The listing builds one solid part. Answer for the finished solid, in the listing's coordinates (mm). Face numbers are marked on the shaded views. A direction names the side the tool comes from. Coordinates: 2 decimals unless noted, no trailing zeros. Loops run counter-clockwise (first coordinate to the right, second up) from the corner with the lowest first, then second, coordinate; pieces in that order, holes last. Notation, with made-up numbers: (79.25, 33.25) - (109.25, 33.25) arc R14 ccw to (109.25, 58.25) - close; hole circle Ø11 at (45.5, 25.5). An arc over 180 degrees is marked (long way). Write each question's results on one line, items separated by ' | '. Start each with the question number.
(1) Consider line 1 (X direction, y = 1, z = 19); line 2 (Z direction, x = 15.5, y = 32); line 3 (Y direction, x = -46.5, z = 54). Determine where each line is inside the solid, lowest interval first. Write a range as from..to.
(2) Determine the mould class of the marked faces 3, 4, 5 and 6 for opening direction X: released by +X, released by -X, zero draft, split by the parting line, or undercut.
(3) Find section C-C on y = -55. Determine the outline of the cut face in (x, z).
(4) Given pin 1 Ø1 at (y, z) = (-42.5, 43) entering from +X; pin 2 Ø23 at (x, z) = (13.5, 28.5) entering from -Y; pin 3 Ø6 at (x, y) = (-2.5, 15) entering from +Z, each flat-ended and moving along its own axis, determine where each tip first touches the part or whether it passes through.
(5) Find section B-B on x = 4. Determine the outline of the cut face in (y, z), then the cut area to 4 significant figures.
(6) For the marked faces 1 and 2, determine the directions among +Z, -Z, +X, -X, +Y, -Y from which every point of the face is accessible in a straight line to the end or side of a thin tool.
from build123d import *

# Parameters (mm, degrees)
PAD_DEPTH    = 80
POCKET_DEPTH = 77
FILLET_R     = 10
FILLET001_R  = 10


with BuildPart() as part:
    # Sketch → Pad (new body)
    with BuildSketch(Plane.XY):
        with BuildLine():
            ThreePointArc((78, -80.5), (83, 0), (78, 80.5))
            Line((78, 80.5), (-78, 80.5))
            ThreePointArc((-78, 80.5), (-84.853217, -2), (-78, -84.5))
            Line((-78, -84.5), (78, -80.5))
        make_face()
    extrude(amount=PAD_DEPTH)

    # Sketch001 (on Face6 of Pad) → Pocket (cut)
    with BuildSketch(Plane.XY.offset(80)):
        with BuildLine():
            Line((-75.633377, -81.450424), (75.073144, -78))
            ThreePointArc((75.073144, -78), (80.164748, 0), (75.073144, 78))
            Line((-75.914692, 78), (75.073144, 78))
            ThreePointArc((-75.914692, 78), (-82.171076, -1.736498), (-75.633377, -81.450424))
        make_face()
    extrude(amount=-POCKET_DEPTH, mode=Mode.SUBTRACT)

    # Fillet
    fillet_edges = [part.edges().sort_by_distance(p)[0] for p in [
        (-75.914692, 78, 41.5),
        (75.073144, 78, 41.5),
        (-75.633377, -81.450424, 41.5),
        (75.073144, -78, 41.5),
    ]]
    fillet(fillet_edges, radius=FILLET_R)

    # Fillet001
    fillet001_edges = [part.edges().sort_by_distance(p)[0] for p in [
        (78, 80.5, 40),
        (78, -80.5, 40),
        (-78, 80.5, 40),
        (-78, -84.5, 40),
    ]]
    fillet(fillet001_edges, radius=FILLET001_R)


solid = part.part
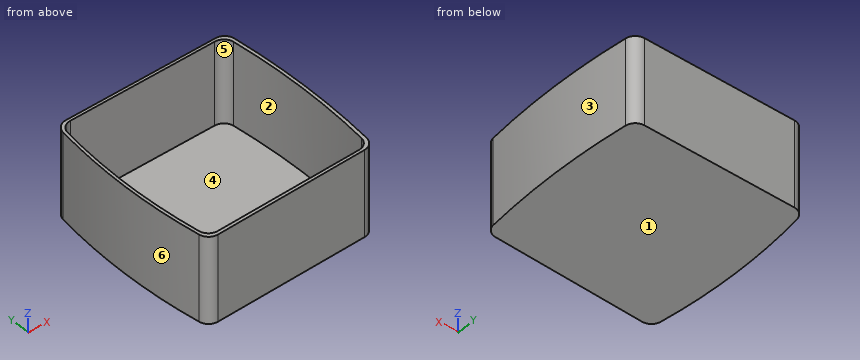
Values:
1) line 1: x = -84.84..-82.17, 80.16..83 | line 2: z = 0..3 | line 3: y = -83.69..-80.78, 78..80.5
2) face 3: released by +X | face 4: undercut | face 5: undercut | face 6: released by -X
3) outline: (-82.04, 0) - (80.67, 0) - (80.67, 80) - (77.64, 80) - (77.64, 3) - (-79.23, 3) - (-79.23, 80) - (-82.04, 80) - close
4) pin 1: stops at x = 81.64 | pin 2: stops at y = -82.45 | pin 3: stops at z = 3
5) outline: (-82.4, 0) - (80.5, 0) - (80.5, 80) - (78, 80) - (78, 3) - (-79.63, 3) - (-79.63, 80) - (-82.4, 80) - close | area: 894.5 mm²
6) face 1: -Z, +X, -X, +Y, -Y | face 2: +Z
